CAD build for the part. Positions are in the model's coordinates, mm. Give positions to 0.01 mm unless a question says otherwise; leave off trailing zeros. Write each loop counter-clockwise with the first axis right and the second up, starting at its lowest first coordinate (ties: lowest second). Pieces come first, ordered by that corner, then holes. Notation, with made-up numbers: (8, 58) -> (60, 58) arc R22 cw to (60, 94) -> close; hole circle Ø8 at (9, 25.5). An arc over 180 degrees is marked (long way). Answer as a JSON object with one key per item and string values.
```python
from build123d import *

# Parameters (mm, degrees)
F0_R     = 12.7
F0_R_2   = 3.81
F1_DEPTH = 3.81


with BuildPart() as f1:
    # F0 (on Top) → F1 (new body, symmetric)
    with BuildSketch(Plane.XY):
        Circle(F0_R)
        Polygon((-9.650616, -7.443798), (-3.955839, -7.81104), (-3.193578, -8.609821), (-8.750626, -8.403624), align=None, mode=Mode.SUBTRACT)
        Polygon((-12.177582, 0.501016), (-8.051188, -3.44084), (-7.980709, -4.542713), (-12.105114, -0.812755), align=None, mode=Mode.SUBTRACT)
        Circle(F0_R_2, mode=Mode.SUBTRACT)
        Polygon((-2.608019, -11.905577), (1.990491, -8.526368), (3.087863, -8.648298), (-1.301624, -12.062344), align=None, mode=Mode.SUBTRACT)
        Polygon((5.654898, -10.796603), (7.005449, -5.252114), (7.924459, -4.64014), (6.756424, -10.076959), align=None, mode=Mode.SUBTRACT)
        Polygon((11.271826, -4.635779), (8.742479, 0.479663), (9.053113, 1.539191), (11.653065, -3.376453), align=None, mode=Mode.SUBTRACT)
        Polygon((-9.033578, 1.649981), (-9.795484, 7.158411), (-9.006522, 8.211399), (-8.379297, 2.539368), align=None, mode=Mode.SUBTRACT)
        Polygon((-1.62121, 12.079578), (-4.78664, 7.331377), (-5.859535, 7.07063), (-2.902438, 11.780077), align=None, mode=Mode.SUBTRACT)
        Polygon((11.614542, 3.694177), (6.388806, 5.987), (5.945714, 6.998317), (11.097108, 4.903933), align=None, mode=Mode.SUBTRACT)
        Polygon((6.522684, 10.295587), (1.04574, 8.692953), (0.05625, 9.182853), (5.348691, 10.889714), align=None, mode=Mode.SUBTRACT)
    extrude(amount=F1_DEPTH, both=True)


solid = f1.part
```
1) Pin check, flat tips, straight feed: pin 1 (2 mm diameter, centred on x = 5, z = -2, fed in from -Y); pin 2 (3 mm diameter, centred on x = 0.5, z = -2.5, fed in from +Y); pin 3 (3 mm diameter, centred on y = -5.5, z = 1.5, fed in from +X). Stop position of each tip, or through.
Model answer:
{"pin 1": "stops at y = -12.05", "pin 2": "stops at y = 12.7", "pin 3": "stops at x = 12.05"}
2) Slice it at D-D (z = -3). State how many separate pieces and enclosed holes the cut face has, then the cut area to 3 significant figures.
Model answer:
{"separate pieces": "1", "enclosed holes": "10", "area": "419 mm2"}
3) Slice it at C-C (y = 9.5). List the corners of the cut face in (x, z), then the cut area to 3 significant figures.
Model answer:
{"outline": "(-8.43, -3.81) -> (-4.33, -3.81) -> (-4.33, 3.81) -> (-8.43, 3.81) -> close; (-3.34, -3.81) -> (1.04, -3.81) -> (1.04, 3.81) -> (-3.34, 3.81) -> close; (3.8, -3.81) -> (8.43, -3.81) -> (8.43, 3.81) -> (3.8, 3.81) -> close", "area": "99.8 mm2"}
4) Mould opens along Y. For faces 1 (the flat face through (3, 3, 3.81)), 2 (the flat face through (2.531, -8.586, 0.053)) say: released by +Y, released by -Y, zero draft, split by the parting line, or undercut.
Model answer:
{"face 1": "zero draft", "face 2": "undercut"}
5) Slice it at A-A (y = -2.25). List the corners of the cut face in (x, z).
Model answer:
{"outline": "(-12.5, -3.81) -> (-10.52, -3.81) -> (-10.52, 3.81) -> (-12.5, 3.81) -> close; (-9.3, -3.81) -> (-3.07, -3.81) -> (-3.07, 3.81) -> (-9.3, 3.81) -> close; (3.07, -3.81) -> (10.09, -3.81) -> (10.09, 3.81) -> (3.07, 3.81) -> close; (11.06, -3.81) -> (12.5, -3.81) -> (12.5, 3.81) -> (11.06, 3.81) -> close"}
6) Wall check: probe 1 along X at (y, z) = (4.25, -1); probe 2 along Y at (x, z) = (-4.25, -0.5); probe 3 along Y at (x, z) = (0, 1). Give the ranges that are in metal, low to high.
Model answer:
{"probe 1": "x = -11.97 to -9.39, -8.57 to 10.35, 11.38 to 11.97", "probe 2": "y = -11.97 to -8.57, -7.79 to 8.14, 9.63 to 11.97", "probe 3": "y = -12.7 to -11.05, -9.99 to -3.81, 3.81 to 12.7"}
7) Slice it at B-B (x = -1). List the corners of the cut face in (y, z).
Model answer:
{"outline": "(-12.66, -3.81) -> (-11.83, -3.81) -> (-11.83, 3.81) -> (-12.66, 3.81) -> close; (-10.72, -3.81) -> (-3.68, -3.81) -> (-3.68, 3.81) -> (-10.72, 3.81) -> close; (3.68, -3.81) -> (12.66, -3.81) -> (12.66, 3.81) -> (3.68, 3.81) -> close"}
